Check sheet for the modelled part. Datum: model origin and axes. Units: mm. A direction names the side the tool comes from. Coordinates: 2 decimals unless noted, no trailing zeros. Loops run counter-clockwise (first coordinate to the right, second up) from the corner with the lowest first, then second, coordinate; pieces in that order, holes last. Notation, with made-up numbers: M 55.25,-0.75 L 114.25,-0.75 A15 cw 114.25,8.25 Z; hole C -5,-17 d4. An arc over 180 degrees is marked long. Answer as CSV lines item,"result". Start each with the question number.
from build123d import *

# Parameters (mm, degrees)
F0_W     = 12.7
F0_H     = 12.7
F1_DEPTH = 30.95625
F2_R     = 6.35
F3_DEPTH = 1.5875
F4_R     = 4.7625
F5_DEPTH = 7.112
F6_W     = 6.35
F6_H     = 28.575
F7_DEPTH = 12.7
F8_R     = 1.7272
F9_DEPTH = 4.7625


with BuildPart() as f1:
    # F0 (on Top) → F1 (new body)
    with BuildSketch(Plane.XY):
        Rectangle(F0_W, F0_H)
    extrude(amount=F1_DEPTH)

    # F2 (on face) → F3 (join)
    with BuildSketch(Plane.XY.offset(30.95625)):
        Circle(F2_R)
    extrude(amount=F3_DEPTH)

    # F4 (on face) → F5 (join)
    with BuildSketch(Plane.XY.offset(32.54375)):
        Circle(F4_R)
    extrude(amount=F5_DEPTH)

    # F6 (on face) → F7 (cut, through all)
    with BuildSketch(Plane(origin=(-6.35, 0, 0), x_dir=(0, -1, 0), z_dir=(-1, 0, 0))):
        with Locations((-3.175, 14.2875)):
            Rectangle(F6_W, F6_H)
    extrude(amount=-F7_DEPTH, mode=Mode.SUBTRACT)

    # F8 (on face) → F9 (cut)
    with BuildSketch(Plane(origin=(0, 0, 0), x_dir=(-1, 0, 0), z_dir=(0, 1, 0))):
        with Locations((0, 23.8125)):
            Circle(F8_R)
        with Locations((0, 4.7625)):
            Circle(F8_R)
    extrude(amount=-F9_DEPTH, mode=Mode.SUBTRACT)


solid = f1.part
Item 1: Material ranges on line 1 (Z direction, x = 0, y = -2.7); line 2 (Z direction, x = -3.5, y = 3) (3 decimals); line 3 (Y direction, x = -4, z = 28.5), recorded low to high. Write a range as from..to.
Item 2: Go/stop test with flat-tipped pins: pin 1 (1.5 mm diameter, centred on x = -5, z = 31, fed in from +Y); pin 2 (1 mm diameter, centred on x = -2, y = -5, fed in from +Z); pin 3 (4 mm diameter, centred on x = 0, z = 5, fed in from +Y); pin 4 (2 mm diameter, centred on x = 0, z = 4.76, fed in from +Y). Record where each tip stops, or that it passes through.
Item 3: Sectioned sample at B-B, the plane x = 3.25. Record the boundary of the cut face in (y, z) (3 decimals), and give its area (3 significant figures).
Item 4: Sectioned sample at C-C, the plane z = 33. Record the boundary of the cut face in (x, y) (1 decimal), and give its area (3 significant figures).
Item 5: Sectioned sample at D-D, the plane y = -2.5. Record the boundary of the cut face in (x, z), and give its area (3 significant figures).
Item 6: Release check for a two-part mould opening along Z. For faces 6 (the face through (0, 3, 28.575)), 7 (the face through (-5, -5, 30.956)), 8 (the face through (0, -4.762, 24)) record: released by +Z, released by -Z, zero draft, split by the parting line, or undercut.
Item 7: Set-up check for faces 1 (the face through (-5, 5, 30.956)), 2 (the face through (5, -5, 30.956)), 3 (the face through (5, 5, 30.956)), 4 (the face through (0, -4.762, 5)), 5 (the face through (-1.38, -6.2, 31.74)): record each of +Z, -Z, +X, -X, +Y, -Y from which the full face is reachable in a straight line by a thin tool's end or side.
Item 8: Sectioned sample at A-A, the plane y = 3.75. Record the boundary of the cut face in (x, z) (3 decimals).
Reply:
1,line 1,"0..3.04, 6.49..22.09, 25.54..39.66"
1,line 2,"28.575..39.656"
1,line 3,"-6.35..0"
2,pin 1,"y = 6.35"
2,pin 2,"z = 32.54"
2,pin 3,"y = 0"
2,pin 4,"y = -4.76"
3,outline,"M -6.35,0 L 0,0 L 0,28.575 L 6.35,28.575 L 6.35,30.956 L 5.455,30.956 L 5.455,32.544 L 3.481,32.544 L 3.481,39.656 L -3.481,39.656 L -3.481,32.544 L -5.455,32.544 L -5.455,30.956 L -6.35,30.956 Z"
3,area,"279 mm²"
4,outline,"C 0,0 d9.5"
4,area,"71.3 mm²"
5,outline,"M -6.35,0 L 6.35,0 L 6.35,30.96 L 5.84,30.96 L 5.84,32.54 L 4.05,32.54 L 4.05,39.66 L -4.05,39.66 L -4.05,32.54 L -5.84,32.54 L -5.84,30.96 L -6.35,30.96 Z; hole C 0,4.76 d3.45; hole C 0,23.81 d3.45"
5,area,"451 mm²"
6,face 6,"released by -Z"
6,face 7,"released by +Z"
6,face 8,"undercut"
7,face 1,"+Z, -X, +Y"
7,face 2,"+Z, +X, -Y"
7,face 3,"+Z, +X, +Y"
7,face 4,"+Y"
7,face 5,"+Z"
8,outline,"M -6.35,28.575 L 6.35,28.575 L 6.35,30.956 L 5.124,30.956 L 5.124,32.544 L 2.936,32.544 L 2.936,39.656 L -2.936,39.656 L -2.936,32.544 L -5.124,32.544 L -5.124,30.956 L -6.35,30.956 Z"
